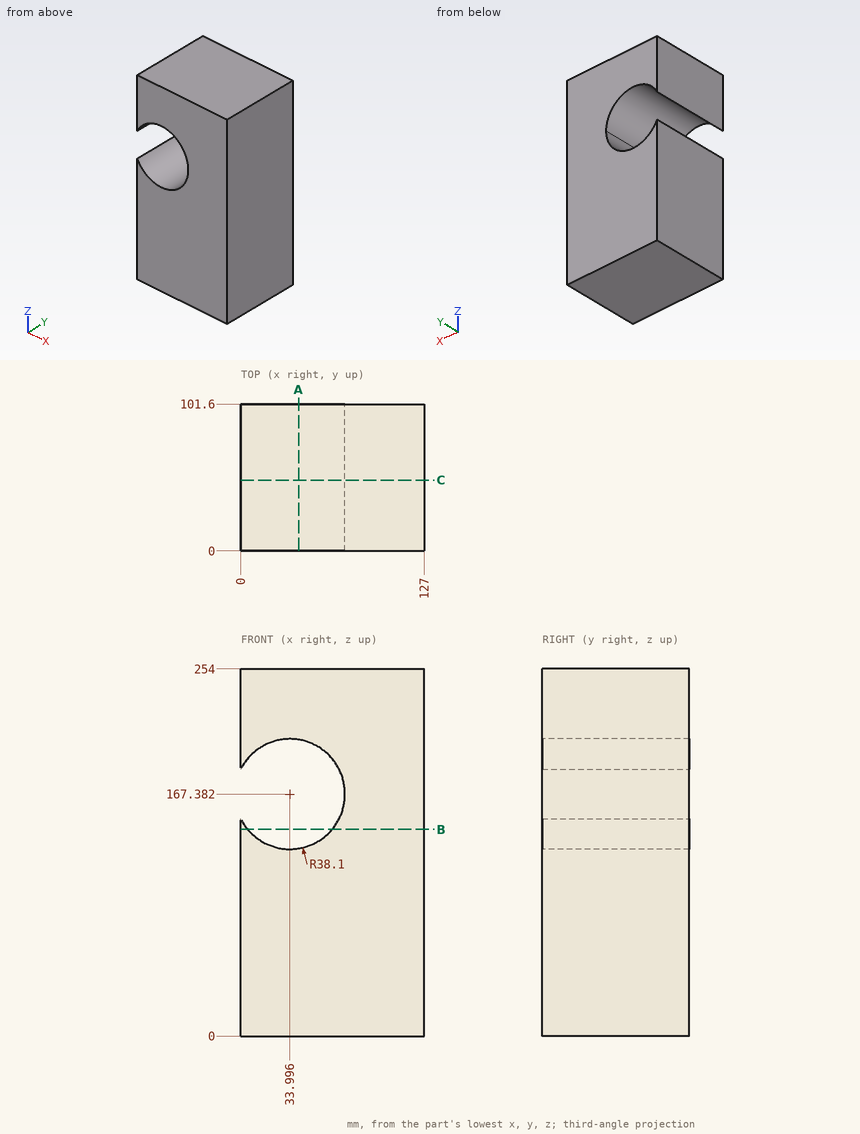
Geometry: see drawing. Coordinates: mm, zero at the bounding-box minimum. Round coordinates to 2 decimals unless told otherwise and drop trailing zeros. Write each loop counter-clockwise with the first axis right and the second up, starting at its lowest first coordinate (ties: lowest second). Pieces come first, ordered by that corner, then holes.
1) Ray query, L1, parallel to X at y = 38.5, z = 195.5 (1 decimal); L2, parallel to Z at x = 23.5, y = 39.5; L3, parallel to Z at x = 37, y = 37.5. Return the intervals inside material, ascending.
2) Cut plane B-B (z = 143). Return the cut outline in (x, y), then the cut area to 3 significant figures.
3) Cut plane C-C (y = 49). Return the cut outline in (x, z) (1 decimal).
4) Cut plane A-A (x = 40). Return the cut outline in (y, z).
Geometry says:
1. L1: x = 0 to 8.3, 59.7 to 127
1. L2: z = 0 to 130.76, 204.01 to 254
1. L3: z = 0 to 129.4, 205.36 to 254
2. outline: (0, 0) - (4.72, 0) - (4.72, 101.6) - (0, 101.6) - close; (63.27, 0) - (127, 0) - (127, 101.6) - (63.27, 101.6) - close
2. area: 6,950 mm2
3. outline: (0, 0) - (127, 0) - (127, 254) - (0, 254) - (0, 184.6) arc R38.1 cw (long way) to (0, 150.2) - close
4. outline: (0, 0) - (101.6, 0) - (101.6, 129.76) - (0, 129.76) - close; (0, 205.01) - (101.6, 205.01) - (101.6, 254) - (0, 254) - close
